CAD build for the part. Positions are in the model's coordinates, mm. A direction names the side the tool comes from. Round coordinates to 2 decimals unless told otherwise and drop trailing zeros. Order: outer loops, then holes, each group sorted by start corner. A loop starts at its lowest first (then second) coordinate and runs counter-clockwise, first axis right, second up. Notation, with made-up numbers: M -10,74 L 1,74 A13 ccw 1,97 Z; hole C 84.5,0 d3. An arc over 180 degrees is marked long. Answer as a JSON object with one key per item and string values.
```python
from build123d import *

# Parameters (mm, degrees)
F2_W     = 0.2083333333
F2_H     = 0.3472222222
F3_DEPTH = 0.2
F4_COUNT = 4


# Not quite as in the source:
# - a feature names something its author has since deleted; it is built from what else it names


with BuildPart() as f1:
    # F0 (on Front) → F1 (revolve)
    with BuildSketch(Plane.XZ):
        with BuildLine():
            Line((0, 14.3055555556), (0, 0))
            Line((0, 0), (0.5729166667, 0))
            Line((0.5729166667, 0), (0.6076388889, 0.2083333333))
            Line((0.6076388889, 0.2083333333), (0.6076388889, 12.7777777778))
            ThreePointArc((0.6076388889, 12.7777777778), (0.5535814562, 13.4119274316), (0.3929690636, 14.0277777778))
            ThreePointArc((0.3929690636, 14.0277777778), (0.2406164888, 14.2290996444), (0, 14.3055555556))
        make_face()
    revolve(axis=Axis((0, 0, 7.1527777778), (0, 0, 1)))

    # F2 (on Front) → F3 (join, symmetric)
    with BuildSketch(Plane.XZ):
        Polygon((0, 10.8660130719), (0, 0.2083333333), (0.6076388889, 0.2083333333), (2.3611111111, 0.2083333333), (2.3611111111, 1.25), (1.5972222222, 1.25), (1.3888888889, 1.25), (0.4, 1.25), (0.4, 1.5972222222), (1.3888888889, 1.5972222222), (1.5972222222, 1.5972222222), (2.3611111111, 1.5972222222), (0.9027777778, 7.6388888889), (0.9027777778, 9.1666666667), align=None)
        with Locations((1.4930555556, 1.4236111111)):
            Rectangle(F2_W, F2_H)
    extrude(amount=F3_DEPTH, both=True)

    # F4: F1 ×4 about axis
    f4_axis = Axis((0, 0, 0.2083333333), (0, 0, 1))


with BuildPart() as f1_1:
    add(f1.part)
    for i in range(1, F4_COUNT):
        add(f1.part.rotate(f4_axis, i * 360 / F4_COUNT))


solid = f1_1.part
```
Item 1: Wall check: line 1 along Y through (x, z) = (-0.95, 5.75); line 2 along X through (y, z) = (0.1, 7.25); line 3 along Y through (x, z) = (-0.35, 10.75). Give the ranges that are in metal, low to high. Write a range as [from, to].
Worked answers:
{"line 1": "y = [-0.2, 0.2]", "line 2": "x = [-1, 1]", "line 3": "y = [-0.5, 0.5]"}
Item 2: Saw through at A-A on y = -1.85. List the corners of the cut face in (x, z).
Worked answers:
{"outline": "M -0.2,0.21 L 0.2,0.21 L 0.2,1.25 L -0.2,1.25 Z; M -0.2,1.6 L 0.2,1.6 L 0.2,3.71 L -0.2,3.71 Z"}
Item 3: Drop a flat-ended pin along its axis: pin 1 Ø1.4 at (x, z) = (-1.5, 3.5) entering from -Y. Give the stop position or say it passes through.
Worked answers:
{"pin 1": "stops at y = -0.2"}
Item 4: Saw through at B-B on z = 1. List the corners of the cut face in (x, y).
Worked answers:
{"outline": "M -2.36,-0.2 L -0.57,-0.2 A0.61 ccw -0.2,-0.57 L -0.2,-2.36 L 0.2,-2.36 L 0.2,-0.57 A0.61 ccw 0.57,-0.2 L 2.36,-0.2 L 2.36,0.2 L 0.57,0.2 A0.61 ccw 0.2,0.57 L 0.2,2.36 L -0.2,2.36 L -0.2,0.57 A0.61 ccw -0.57,0.2 L -2.36,0.2 Z"}
Item 5: 3-axis set-ups, long thin cutter, end or side, ignore diameter. For faces 1 (the flat face through (0.2, 1, 4)), 2 (the flat face through (1, -0.2, 4)), 3 (the flat face through (-1, 0.2, 4)): which of +Z, -Z, +X, -X, +Y, -Y reach the whole face in a straight line?
Worked answers:
{"face 1": "+Z, -Z, +X, +Y", "face 2": "+Z, -Z, +X, -Y", "face 3": "+Z, -Z, -X, +Y"}
Item 6: Saw through at C-C on y = 1.1. List the corners of the cut face in (x, z).
Worked answers:
{"outline": "M -0.2,0.21 L 0.2,0.21 L 0.2,1.25 L -0.2,1.25 Z; M -0.2,1.6 L 0.2,1.6 L 0.2,6.82 L -0.2,6.82 Z"}
Item 7: Saw through at D-D on x = 0. State how many separate pieces and enclosed holes the cut face has, and give its area (3 significant figures).
Worked answers:
{"separate pieces": "1", "enclosed holes": "2", "area": "34.3 mm2"}
